from build123d import *

# Parameters (mm, degrees)
BOSS_EXTRUDE1_DEPTH = 9
SKETCH2_R           = 2
BOSS_EXTRUDE2_DEPTH = 4
SKETCH3_W           = 13
SKETCH3_H           = 13
BOSS_EXTRUDE3_DEPTH = 55


with BuildPart() as part:
    # Sketch1 → Boss-Extrude1 (new, symmetric)
    with BuildSketch(Plane(origin=(0, 0, 0), x_dir=(0, 0, -1), z_dir=(1, 0, 0))):
        Polygon((-26.5, 10), (26.5, 10), (26.5, -7), (17.5, -7), (17.5, -10), (-26.5, -10), align=None)
    extrude(amount=BOSS_EXTRUDE1_DEPTH, both=True)

    # Sketch2 → Boss-Extrude2 (add, symmetric)
    with BuildSketch(Plane(origin=(0, 0, 0), x_dir=(0, 0, -1), z_dir=(1, 0, 0))):
        with BuildLine():
            Line((-31.5, 7), (-26.5, 7))
            Line((-26.5, 7), (-26.5, -3))
            Line((-26.5, -3), (-31.5, -3))
            ThreePointArc((-31.5, -3), (-36.5, 2), (-31.5, 7))
        make_face()
        with Locations((-31.5, 2)):
            Circle(SKETCH2_R, mode=Mode.SUBTRACT)
    extrude(amount=BOSS_EXTRUDE2_DEPTH, both=True)

    # Sketch3 → Boss-Extrude3 (add)
    with BuildSketch(Plane(origin=(0, 0, -26.5), x_dir=(-1, 0, 0), z_dir=(0, 0, -1))):
        with Locations((0, 1.5)):
            Rectangle(SKETCH3_W, SKETCH3_H)
    extrude(amount=BOSS_EXTRUDE3_DEPTH)


solid = part.part
Source: CAD feature listing. Evaluate the final solid. Frame: model axes, mm. A direction names the side the tool comes from. Give positions to 0.01 mm unless a question says otherwise; leave off trailing zeros. Order: outer loops, then holes, each group sorted by start corner. A loop starts at its lowest first (then second) coordinate and runs counter-clockwise, first axis right, second up. Notation, with made-up numbers: (-25, -29) -> (-6, -29) arc R28 cw to (-6, 5) -> close; hole circle Ø4 at (86, 34.5). An arc over 180 degrees is marked (long way). Write item = value, one per line.
Q1. Pin query (flat end, axial travel): pin 1 (4 mm diameter, centred on x = -1, z = 29, fed in from -Y); pin 2 (8 mm diameter, centred on y = -4.5, z = -50.5, fed in from -X); pin 3 (4 mm diameter, centred on x = 1.5, z = -46, fed in from -Y). Return the tip coordinate at first contact, or that it passes through.
Data:
pin_1 = -3
pin_2 = -6.5
pin_3 = -5
Q2. Cut plane B-B, the plane x = 2.75. Output: boundary loops of the cut face in (y, z).
Data:
outline = (-10, -17.5) -> (-7, -17.5) -> (-7, -26.5) -> (-5, -26.5) -> (-5, -81.5) -> (8, -81.5) -> (8, -26.5) -> (10, -26.5) -> (10, 26.5) -> (7, 26.5) -> (7, 31.5) arc R5 ccw to (-3, 31.5) -> (-3, 26.5) -> (-10, 26.5) -> close; hole circle Ø4 at (2, 31.5)
Q3. Material intervals for line 1 (Y direction, x = -2.25, z = 31.5); line 2 (Z direction, x = -2, y = 1.75); line 3 (Y direction, x = -2, z = -32), sorted ascending. Write a range as from..to.
Data:
line_1 = -3..0, 4..7
line_2 = -81.5..29.52, 33.48..36.49
line_3 = -5..8
Q4. Cut plane C-C, the plane x = 7.75. Output: boundary loops of the cut face in (y, z), and give its area (3 significant figures).
Data:
outline = (-10, -17.5) -> (-7, -17.5) -> (-7, -26.5) -> (10, -26.5) -> (10, 26.5) -> (-10, 26.5) -> close
area = 1,030 mm^2
Q5. Cut plane D-D, the plane y = -8.5. Output: boundary loops of the cut face in (x, z).
Data:
outline = (-9, -17.5) -> (9, -17.5) -> (9, 26.5) -> (-9, 26.5) -> close
Q6. Pull-direction query (Z, two-part tool) for faces 4 (the face through (0, -8, -17.5)), 5 (the face through (0, -7, -22)), 6 (the face through (-0.056, 2.601, 29.592)), 7 (the face through (0.1, 1.9, 36.5)); classes: released by +Z, released by -Z, zero draft, split by the parting line, or undercut.
Data:
face_4 = released by -Z
face_5 = zero draft
face_6 = undercut
face_7 = released by +Z
Q7. Cut plane A-A, the plane y = 2. Output: boundary loops of the cut face in (x, z).
Data:
outline = (-9, -26.5) -> (-6.5, -26.5) -> (-6.5, -81.5) -> (6.5, -81.5) -> (6.5, -26.5) -> (9, -26.5) -> (9, 26.5) -> (4, 26.5) -> (4, 29.5) -> (-4, 29.5) -> (-4, 26.5) -> (-9, 26.5) -> close; (-4, 33.5) -> (4, 33.5) -> (4, 36.5) -> (-4, 36.5) -> close
Q8. Set-up query: faces 1 (the face through (6.5, 1, -54)), 2 (the face through (0, 8, -54)), 3 (the face through (4, 2, 29)). Return all of +Z, -Z, +X, -X, +Y, -Y with unobstructed straight access to the full face (end or side cutting, diameter ignored); none if empty.
Data:
face_1 = -Z, +X, +Y, -Y
face_2 = -Z, +X, -X, +Y
face_3 = +Z, +X, +Y, -Y
